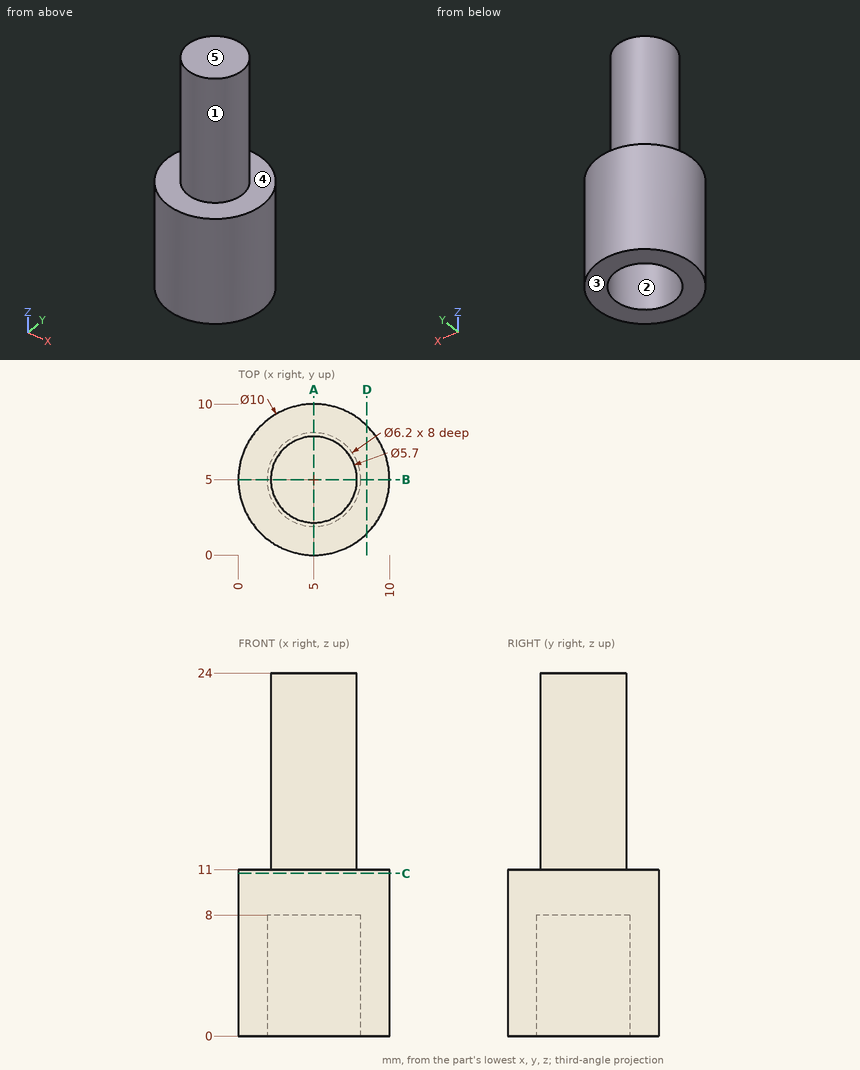
Here's the drawing with two shaded views (mm, measured from the low corner). I have some questions. A direction names the side the tool comes from. Give positions to 0.01 mm unless a question says otherwise; leave off trailing zeros. Loops run counter-clockwise (first coordinate to the right, second up) from the corner with the lowest first, then second, coordinate; pieces in that order, holes last. Notation, with made-up numbers: (37.25, 21) - (79.25, 21) arc R34 ccw to (79.25, 54) - close; hole circle Ø11 at (79.5, 72.25). An arc over 180 degrees is marked (long way). Answer in a Markdown table with one row per item. Add a question column.
Q1. For pin 1 (3 mm diameter, centred on x = 7.5, z = 16, fed in from +Y); pin 2 (1.5 mm diameter, centred on x = 4.5, z = 16, fed in from -Y); pin 3 (5 mm diameter, centred on y = 5, z = 14.5, fed in from -X), each with a flat end and sliding along its axis, tell me the tip position at first contact or that it passes through.
Q2. Please list where these lines run through material, in increasing order: L1, parallel to Y at x = 5, z = 4; L2, parallel to Z at x = 6.25, y = 3.5; L3, parallel to Z at x = 1.5, y = 4.25. Write a range as from..to.
Q3. Which directions (+Z, -Z, +X, -X, +Y, -Y) give clear straight access to the entire face, cutting with the end or side of a thin tool? Please do the marked faces 4 and 5.
Q4. If we section it at A-A (x = 5): List the corners of the cut face in (y, z) for me.
Q5. We'd pull the mould along X, two halves only. Please class the marked faces 1, 2 and 3: +X half, -X half, draft (parallel to the pull), parting line (faces both ways), or undercut.
Q6. If we section it at D-D (x = 8.5): List the corners of the cut face in (y, z) for me, plus the area to 3 significant figures.
Q7. If we section it at C-C (z = 10.75): List the corners of the cut face in (x, y) for me.
The answers:
| question | item | result |
|---|---|---|
| 1 | pin 1 | stops at y = 7.67 |
| 1 | pin 2 | stops at y = 2.15 |
| 1 | pin 3 | stops at x = 2.15 |
| 2 | L1 | y = 0..1.9, 8.1..10 |
| 2 | L2 | z = 8..24 |
| 2 | L3 | z = 0..11 |
| 3 | face 4 | +Z |
| 3 | face 5 | +Z, +X, -X, +Y, -Y |
| 4 | outline | (0, 0) - (1.9, 0) - (1.9, 8) - (8.1, 8) - (8.1, 0) - (10, 0) - (10, 11) - (7.85, 11) - (7.85, 24) - (2.15, 24) - (2.15, 11) - (0, 11) - close |
| 5 | face 1 | parting line |
| 5 | face 2 | undercut |
| 5 | face 3 | draft |
| 6 | outline | (1.43, 0) - (8.57, 0) - (8.57, 11) - (1.43, 11) - close |
| 6 | area | 78.6 mm^2 |
| 7 | outline | circle Ø10 at (5, 5) |
